Source: CAD feature listing. Evaluate the final solid. Frame: model axes, mm. Coordinates: 2 decimals unless noted, no trailing zeros. Loops run counter-clockwise (first coordinate to the right, second up) from the corner with the lowest first, then second, coordinate; pieces in that order, holes last.
```python
from build123d import *

# Parameters (mm, degrees)
MAINBODY_EXTRUDE_START = -90
PROJECTIONXY_SKETCH_W  = 30
PROJECTIONXY_SKETCH_H  = 70
MAINBODY_EXTRUDE_DEPTH = 180
TROUGH_CUT_DEPTH       = 98.724101428
TROUGH_CUT_DEPTH_BACK  = 98.724101428
TROUGH_SKETCH_W        = 10.514570696
TROUGH_SKETCH_H        = 10.514570696


with BuildPart() as part:
    # projectionXy_sketch → mainBody_extrude (new body)
    with BuildSketch(Plane.XY.offset(MAINBODY_EXTRUDE_START)):
        Rectangle(PROJECTIONXY_SKETCH_W, PROJECTIONXY_SKETCH_H)
    extrude(amount=MAINBODY_EXTRUDE_DEPTH)

    # trough_sketch → trough_cut (cut, two sides: drawn at the far end of the back side and taken through both)
    with BuildSketch(Plane(origin=(0, 0, 0), x_dir=(1, 0, 0), z_dir=(0, 0, -1)).offset(-TROUGH_CUT_DEPTH_BACK)):
        with Locations((0, 29.742714652)):
            Rectangle(TROUGH_SKETCH_W, TROUGH_SKETCH_H)
    extrude(amount=TROUGH_CUT_DEPTH + TROUGH_CUT_DEPTH_BACK, mode=Mode.SUBTRACT)


solid = part.part
```
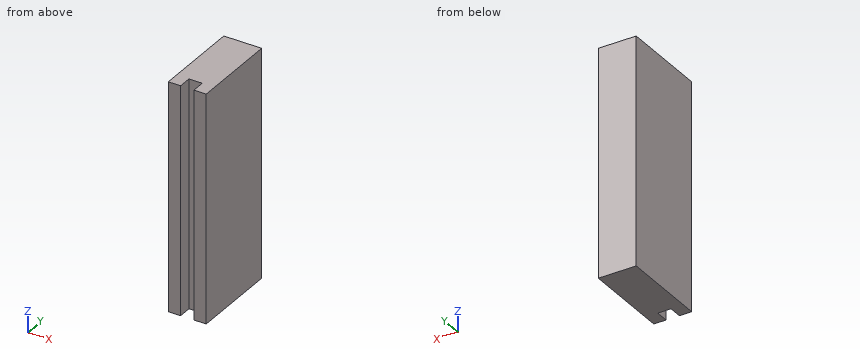
Q1. Section query B-B on z = 35. Return the cut outline in (x, y), then the cut area to 3 significant figures.
Q2. First-contact query: pin 1 Ø8.5 at (x, z) = (-1.5, -5) entering from -Y. Flat tip, straight axial feed; report the tip coordinate or a pass-through.
Q3. Material intervals for line 1 along X through (y, z) = (-28, -79); line 2 along Y through (x, z) = (2, -55), sorted ascending.
Q4. Section query C-C on x = 1.25. Return the cut outline in (y, z), then the cut area to 3 significant figures.
Q5. Section query A-A on y = -28.5. Return the cut outline in (x, z).
Resolved:
1. outline: (-15, -35) - (-5.26, -35) - (-5.26, -24.49) - (5.26, -24.49) - (5.26, -35) - (15, -35) - (15, 35) - (-15, 35) - close
1. area: 1,990 mm2
2. pin 1: stops at y = -35
3. line 1: x = -15 to -5.26, 5.26 to 15
3. line 2: y = -24.49 to 35
4. outline: (-24.49, -90) - (35, -90) - (35, 90) - (-24.49, 90) - close
4. area: 10,700 mm2
5. outline: (-15, -90) - (-5.26, -90) - (-5.26, 90) - (-15, 90) - close; (5.26, -90) - (15, -90) - (15, 90) - (5.26, 90) - close
